```python
from build123d import *

# Parameters (mm, degrees)
SKETCH1_W           = 50.8
SKETCH1_H           = 38.1
BOSS_EXTRUDE1_DEPTH = 6.35
SKETCH2_R           = 6.35
BOSS_EXTRUDE2_DEPTH = 12.7


with BuildPart() as part:
    # Sketch1 → Boss-Extrude1 (new body)
    with BuildSketch(Plane(origin=(0, 0, 0), x_dir=(1, 0, 0), z_dir=(0, 1, 0))):
        with Locations((25.4, 19.05)):
            Rectangle(SKETCH1_W, SKETCH1_H)
    extrude(amount=BOSS_EXTRUDE1_DEPTH)

    # Sketch2 → Boss-Extrude2 (add)
    with BuildSketch(Plane(origin=(0, 6.35, 0), x_dir=(1, 0, 0), z_dir=(0, 1, 0))):
        with Locations(Location((25.4, 19.05, 0), (0, 0, 270))):
            Circle(SKETCH2_R)
        with BuildLine():
            Line((23.570219541, 16.9926), (27.229780459, 16.9926))
            ThreePointArc((27.229780459, 16.9926), (25.4, 21.80336), (23.570219541, 16.9926))
        make_face(mode=Mode.SUBTRACT)
    extrude(amount=BOSS_EXTRUDE2_DEPTH)


solid = part.part
```
Work out the finished part from the listing and answer in its coordinate system (mm). A direction names the side the tool comes from. Give positions to 0.01 mm unless a question says otherwise; leave off trailing zeros. Order: outer loops, then holes, each group sorted by start corner. A loop starts at its lowest first (then second) coordinate and runs counter-clockwise, first axis right, second up. Notation, with made-up numbers: (-28, 21.25) - (31, 21.25) arc R34 ccw to (31, 57.25) - close; hole circle Ø6 at (66.25, 73). An arc over 180 degrees is marked (long way). One line per item, written item: value. Start each with the question number.
1. For a pull along Z with two mould halves and no side action, classify faces 3 (the face through (25, 6.35, -19)), 4 (the face through (25, 3, 0)), 5 (the face through (25, 19.05, -16)) as released by +Z, released by -Z, zero draft, split by the parting line, or undercut.
2. Section D-D, the plane x = 12.5 is taken. Write down the section's boundary in (y, z), then the cut area to 3 significant figures.
3. Section B-B, the plane y = 13 is taken. Write down the section's boundary in (x, z), then the cut area to 3 significant figures.
4. Each of these flat-tipped pins is pushed along its axis until it touches: pin 1 Ø4 at (y, z) = (16.5, -10) entering from +X; pin 2 Ø5.5 at (x, z) = (25.5, -19.5) entering from +Y; pin 3 Ø3 at (x, y) = (25.5, 12.5) entering from -Z; pin 4 Ø6 at (y, z) = (12.5, -15) entering from +X. Where does it stop, or does it pass through?
5. Section A-A, the plane x = 25.4 is taken. Write down the section's boundary in (y, z), then the cut area to 3 significant figures.
6. Section C-C, the plane z = -19.05 is taken. Write down the section's boundary in (x, y), then the cut area to 3 significant figures.
7. Consider line 1 (X direction, y = 11.25, z = -19.05); line 2 (Z direction, x = 25.5, y = 14.25); line 3 (Y direction, x = 34, z = -23). Determine where each line is inside the solid, lowest interval first.
8. Which of the six approach directions +Z, -Z, +X, -X, +Y, -Y give full straight-line access (tool end or side, diameter ignored) to faces 1 (the face through (25, 3, -38.1)), 2 (the face through (31, 6.35, -24))?
Filled sheet:
1. face 3: undercut
1. face 4: released by +Z
1. face 5: zero draft
2. outline: (0, -38.1) - (6.35, -38.1) - (6.35, 0) - (0, 0) - close
2. area: 242 mm²
3. outline: circle Ø12.7 at (25.4, -19.05); hole (23.57, -16.99) arc R2.75 ccw (long way) to (27.23, -16.99) - close
3. area: 105 mm²
4. pin 1: through
4. pin 2: y = 19.05
4. pin 3: z = -25.4
4. pin 4: x = 31.66
5. outline: (0, -38.1) - (6.35, -38.1) - (6.35, -25.4) - (19.05, -25.4) - (19.05, -21.8) - (6.35, -21.8) - (6.35, -16.99) - (19.05, -16.99) - (19.05, -12.7) - (6.35, -12.7) - (6.35, 0) - (0, 0) - close
5. area: 342 mm²
6. outline: (0, 0) - (50.8, 0) - (50.8, 6.35) - (31.75, 6.35) - (31.75, 19.05) - (28.15, 19.05) - (28.15, 6.35) - (22.65, 6.35) - (22.65, 19.05) - (19.05, 19.05) - (19.05, 6.35) - (0, 6.35) - close
6. area: 414 mm²
7. line 1: 19.05 to 22.65, 28.15 to 31.75
7. line 2: -25.4 to -21.8, -16.99 to -12.7
7. line 3: 0 to 6.35
8. face 1: -Z, +X, -X, +Y, -Y
8. face 2: +Y
